Verification items for the finished model (mm, model axes). Face numbers are marked on the shaded views. A direction names the side the tool comes from. Give positions to 0.01 mm unless a question says otherwise; leave off trailing zeros. Loops run counter-clockwise (first coordinate to the right, second up) from the corner with the lowest first, then second, coordinate; pieces in that order, holes last. Notation, with made-up numbers: (-23.75, 68.5) - (17.25, 68.5) arc R27 ccw to (17.25, 105.5) - close; hole circle Ø7 at (-14, 74). An arc over 180 degrees is marked (long way). Put each result on its own line as item: value. Start each with the question number.
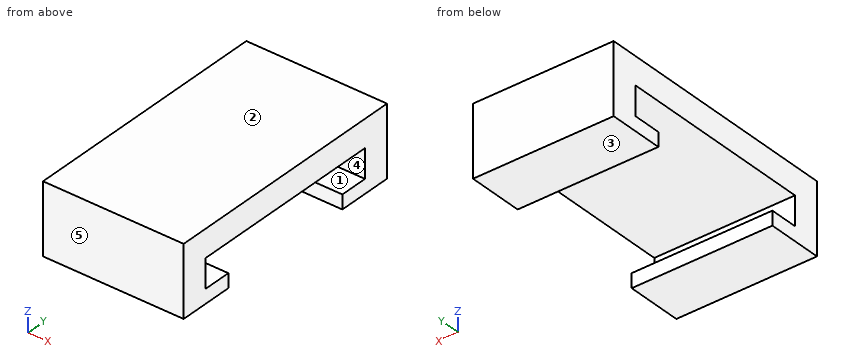
```python
from build123d import *

# Parameters (mm, degrees)
F0_W     = 10
F0_H     = 18
F1_DEPTH = 5
F3_DEPTH = 10.001


with BuildPart() as f1:
    # F0 (on Top) → F1 (new body)
    with BuildSketch(Plane.XY):
        Rectangle(F0_W, F0_H)
    extrude(amount=F1_DEPTH)

    # F2 (on face) → F3 (cut, through all)
    with BuildSketch(Plane.YZ.offset(5)):
        Polygon((-5.05, 1), (-5.05, 0), (5.05, 0), (5.05, 1), (7.05, 1), (7.05, 3.05), (-7.05, 3.05), (-7.05, 1), align=None)
    extrude(amount=-F3_DEPTH, mode=Mode.SUBTRACT)


solid = f1.part
```
1) Section check B-B, the plane y = -6. Enter the section's corners in (x, z).
2) Scan lines: line 1 along Y through (x, z) = (2.5, 2); line 2 along Y through (x, z) = (4.75, 0.4); line 3 along Z through (x, y) = (1.5, 3). Record each from-to range of solid material in increasing order. Write a range as from..to.
3) Draft check along Y on the marked faces 3, 4 and 5. Enter one of: pulls with the +Y half, pulls with the -Y half, needs draft (parallel to the pull), parting line crosses it, or undercut.
4) Section check D-D, the plane y = 1.25. Enter the section's corners in (x, z).
5) Set-up check for the marked faces 1 and 2: record each of +Z, -Z, +X, -X, +Y, -Y from which the full face is reachable in a straight line by a thin tool's end or side.
6) Depth check by flat-ended pin: P1, Ø1.5, axis at y = 1.5, z = 1.5, coming from the -X side; P2, Ø3, axis at x = 1, y = -1.5, coming from the -Z side. Enter the tip coordinate at first touch or a pass-through.
7) Section check A-A, the plane z = 2.35. Enter the section's corners in (x, y), plus the area to 3 significant figures.
8) Section check C-C, the plane x = 4.5. Enter the section's corners in (y, z).
Results are:
1. outline: (-5, 0) - (5, 0) - (5, 1) - (-5, 1) - close; (-5, 3.05) - (5, 3.05) - (5, 5) - (-5, 5) - close
2. line 1: y = -9..-7.05, 7.05..9
2. line 2: y = -9..-5.05, 5.05..9
2. line 3: z = 3.05..5
3. face 3: needs draft
3. face 4: undercut
3. face 5: pulls with the -Y half
4. outline: (-5, 3.05) - (5, 3.05) - (5, 5) - (-5, 5) - close
5. face 1: +X, -X
5. face 2: +Z, +X, -X, +Y, -Y
6. P1: passes through
6. P2: stops at z = 3.05
7. outline: (-5, -9) - (5, -9) - (5, -7.05) - (-5, -7.05) - close; (-5, 7.05) - (5, 7.05) - (5, 9) - (-5, 9) - close
7. area: 39.0 mm2
8. outline: (-9, 0) - (-5.05, 0) - (-5.05, 1) - (-7.05, 1) - (-7.05, 3.05) - (7.05, 3.05) - (7.05, 1) - (5.05, 1) - (5.05, 0) - (9, 0) - (9, 5) - (-9, 5) - close
